from build123d import *

# Parameters (mm, degrees)
SKETCH1_W           = 180
SKETCH1_H           = 45
BOSS_EXTRUDE1_DEPTH = 3.175
FILLET1_R           = 5
SKETCH4_R           = 3
SKETCH4_R_2         = 1.5
CUT_EXTRUDE1_DEPTH  = 157.65672863
SKETCH5_R           = 4
CUT_EXTRUDE2_DEPTH  = 157.65672863
SKETCH6_R           = 1.5
SKETCH6_R_2         = 11.5
CUT_EXTRUDE3_DEPTH  = 157.65672863
SKETCH10_R          = 1.5
CUT_EXTRUDE4_DEPTH  = 157.65672863


with BuildPart() as part:
    # Sketch1 → Boss-Extrude1 (new body)
    with BuildSketch(Plane(origin=(0, 0, 0), x_dir=(1, 0, 0), z_dir=(0, 1, 0))):
        with Locations((65, 0)):
            Rectangle(SKETCH1_W, SKETCH1_H)
    extrude(amount=BOSS_EXTRUDE1_DEPTH)

    # Fillet1
    fillet1_edges = [part.edges().sort_by_distance(p)[0] for p in [
        (-25, 1.5875, -22.5),
        (155, 1.5875, -22.5),
        (155, 1.5875, 22.5),
        (-25, 1.5875, 22.5),
    ]]
    fillet(fillet1_edges, radius=FILLET1_R)

    # Sketch4 → Cut-Extrude1 (cut, through all)
    with BuildSketch(Plane(origin=(0, 3.175, 0), x_dir=(1, 0, 0), z_dir=(0, 1, 0))):
        with Locations(Location((130, 0, 0), (0, 0, 270))):
            Circle(SKETCH4_R)
        with Locations(Location((116, 9, 0), (0, 0, 270))):
            Circle(SKETCH4_R_2)
        with Locations(Location((144, 9, 0), (0, 0, 90))):
            Circle(SKETCH4_R_2)
        with Locations(Location((144, -9, 0), (0, 0, 270))):
            Circle(SKETCH4_R_2)
        with Locations(Location((116, -9, 0), (0, 0, 90))):
            Circle(SKETCH4_R_2)
    extrude(amount=-CUT_EXTRUDE1_DEPTH, mode=Mode.SUBTRACT)

    # Sketch5 → Cut-Extrude2 (cut, through all)
    with BuildSketch(Plane(origin=(0, 3.175, 0), x_dir=(1, 0, 0), z_dir=(0, 1, 0))):
        with Locations(Location((0, 0, 0), (0, 0, 270))):
            Circle(SKETCH5_R)
    extrude(amount=-CUT_EXTRUDE2_DEPTH, mode=Mode.SUBTRACT)

    # Sketch6 → Cut-Extrude3 (cut, through all)
    with BuildSketch(Plane(origin=(0, 3.175, 0), x_dir=(1, 0, 0), z_dir=(0, 1, 0))):
        with Locations(Location((14.5, -15.5, 0), (0, 0, 270))):
            Circle(SKETCH6_R)
        with Locations(Location((14.5, 15.5, 0), (0, 0, 90))):
            Circle(SKETCH6_R)
        with Locations(Location((45.5, 15.5, 0), (0, 0, 270))):
            Circle(SKETCH6_R)
        with Locations(Location((45.5, -15.5, 0), (0, 0, 90))):
            Circle(SKETCH6_R)
        with Locations(Location((30, 0, 0), (0, 0, 270))):
            Circle(SKETCH6_R_2)
    extrude(amount=-CUT_EXTRUDE3_DEPTH, mode=Mode.SUBTRACT)

    # Sketch10 → Cut-Extrude4 (cut, through all)
    with BuildSketch(Plane(origin=(0, 3.175, 0), x_dir=(1, 0, 0), z_dir=(0, 1, 0))):
        with Locations(Location((65.5, -17.5, 0), (0, 0, 270))):
            Circle(SKETCH10_R)
        with Locations(Location((96, -17.5, 0), (0, 0, 270))):
            Circle(SKETCH10_R)
        with Locations(Location((96, 17.5, 0), (0, 0, 90))):
            Circle(SKETCH10_R)
        with Locations(Location((65.5, 17.5, 0), (0, 0, 90))):
            Circle(SKETCH10_R)
    extrude(amount=-CUT_EXTRUDE4_DEPTH, mode=Mode.SUBTRACT)


solid = part.part
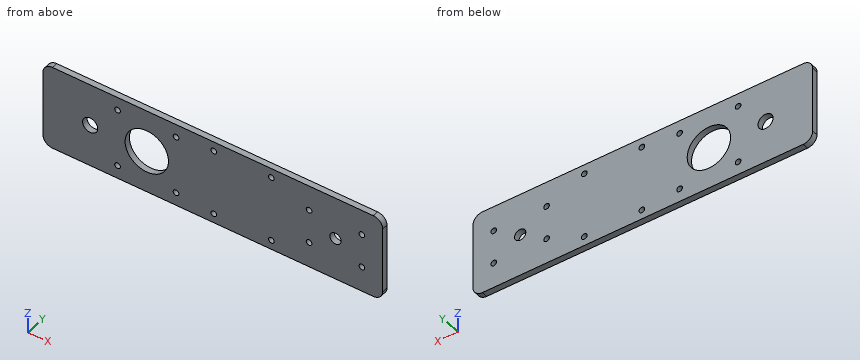
Model file for the job. Use its own axes, mm. Coordinates: 2 decimals unless noted, no trailing zeros. Write each loop counter-clockwise with the first axis right and the second up, starting at its lowest first coordinate (ties: lowest second). Pieces come first, ordered by that corner, then holes. Notation, with made-up numbers: (-33.5, 19) - (-10.5, 19) arc R22 cw to (-10.5, 57) - close; hole circle Ø4 at (-8, -23). An arc over 180 degrees is marked (long way). Write each question's results on one line, items separated by ' | '. Start each with the question number.
1) Cut at B-B (y = 0.95). Count the separate pieces of the cut face and the enclosed holes in it, then the cut area to 3 significant figures.
2) Cut at A-A (x = 14.5). Write the cut outline in (y, z) (3 decimals), then the cut area to 3 significant figures.
3) Cut at D-D (z = 9). Write the cut outline in (x, y) (3 decimals), then the cut area to 3 significant figures.
4) Probe line 1 along X through (y, z) = (1.15, 15.5); line 2 along Z through (x, y) = (96, 2.55); line 3 along Z through (x, y) = (116, 1). List the from-to ranges inside material, lowest first. Write a range as from..to.
5) Cut at C-C (x = 130). Write the cut outline in (y, z) (3 decimals), then the cut area to 3 significant figures.
6) Flat gauge pin, fed straight in: P1, Ø2.5, axis at x = 116, z = 9, coming from the -Y side. Where does the tip first touch, or does it go through?
Returned:
1) separate pieces: 1 | enclosed holes: 15 | area: 7,500 mm^2
2) outline: (0, -22.5) - (3.175, -22.5) - (3.175, -17) - (0, -17) - close; (0, -14) - (3.175, -14) - (3.175, 14) - (0, 14) - close; (0, 17) - (3.175, 17) - (3.175, 22.5) - (0, 22.5) - close | area: 124 mm^2
3) outline: (-25, 0) - (22.841, 0) - (22.841, 3.175) - (-25, 3.175) - close; (37.159, 0) - (114.5, 0) - (114.5, 3.175) - (37.159, 3.175) - close; (117.5, 0) - (142.5, 0) - (142.5, 3.175) - (117.5, 3.175) - close; (145.5, 0) - (155, 0) - (155, 3.175) - (145.5, 3.175) - close | area: 507 mm^2
4) line 1: -25..13, 16..44, 47..155 | line 2: -22.5..-19, -16..16, 19..22.5 | line 3: -22.5..-10.5, -7.5..7.5, 10.5..22.5
5) outline: (0, -22.5) - (3.175, -22.5) - (3.175, -3) - (0, -3) - close; (0, 3) - (3.175, 3) - (3.175, 22.5) - (0, 22.5) - close | area: 124 mm^2
6) P1: through
